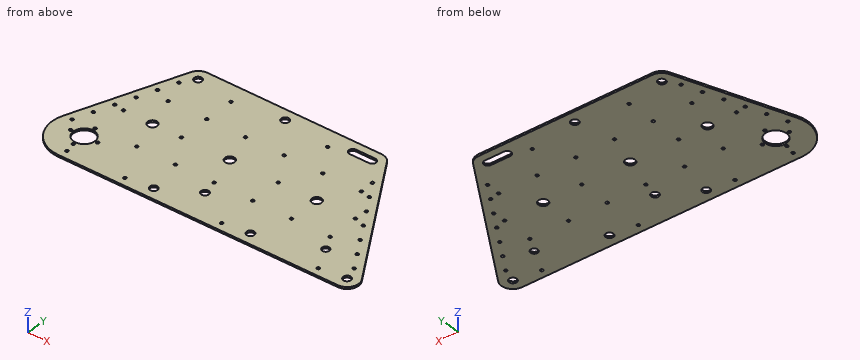
from build123d import *

# Parameters (mm, degrees)
SKETCH2_R           = 3.9998
SKETCH2_R_2         = 1.499925
SKETCH2_R_3         = 4.99975
SKETCH2_R_4         = 3.7498125
SKETCH2_R_5         = 1.5
SKETCH2_R_6         = 10.99945
BOSS_EXTRUDE1_DEPTH = 2


with BuildPart() as part:
    # Sketch2 → Boss-Extrude1 (new body)
    with BuildSketch(Plane.XY):
        with BuildLine():
            Line((96.362607148, 83.91244893), (182.746139217, -55.124360407))
            ThreePointArc((182.746139217, -55.124360407), (183.120738534, -67.267781048), (172.665833933, -73.456315551))
            Line((172.665833933, -73.456315551), (-116.301106221, -73.709344442))
            ThreePointArc((-116.301106221, -73.709344442), (-143.610306979, -59.428306601), (-147.408355202, -28.84538134))
            Line((-147.408355202, -28.84538134), (-105.239440592, 83.486872373))
            ThreePointArc((-105.239440592, 83.486872373), (-100.811651195, 88.586021375), (-94.331273913, 90.486376541))
            Line((-94.331273913, 90.486376541), (85.638662445, 90.486376541))
            ThreePointArc((85.638662445, 90.486376541), (91.93104468, 88.717175744), (96.362607148, 83.91244893))
        make_face()
        with Locations((-94.331273913, 78.486872372)):
            Circle(SKETCH2_R, mode=Mode.SUBTRACT)
        with Locations((-4.335773913, 78.486872372)):
            Circle(SKETCH2_R, mode=Mode.SUBTRACT)
        with Locations((-54.333273913, 70.986872372)):
            Circle(SKETCH2_R_2, mode=Mode.SUBTRACT)
        with Locations((-103.671855402, 65.368244598)):
            Circle(SKETCH2_R_2, mode=Mode.SUBTRACT)
        with Locations((-110.669996254, 46.632415776)):
            Circle(SKETCH2_R_2, mode=Mode.SUBTRACT)
        with Locations((-94.331273913, 39.98689418)):
            Circle(SKETCH2_R_2, mode=Mode.SUBTRACT)
        with Locations((-117.667881298, 27.897271817)):
            Circle(SKETCH2_R_2, mode=Mode.SUBTRACT)
        with Locations((-114.330273913, 7.486872372)):
            Circle(SKETCH2_R_2, mode=Mode.SUBTRACT)
        with Locations((-124.665791603, 9.162060229)):
            Circle(SKETCH2_R_2, mode=Mode.SUBTRACT)
        with Locations((-131.663765383, -9.573321299)):
            Circle(SKETCH2_R_2, mode=Mode.SUBTRACT)
        with Locations((-116.330173913, -26.513127628)):
            Circle(SKETCH2_R_2, mode=Mode.SUBTRACT)
        with Locations((-138.661805034, -28.308879181)):
            Circle(SKETCH2_R_2, mode=Mode.SUBTRACT)
        with Locations((-130.329473913, -40.513127628)):
            Circle(SKETCH2_R_2, mode=Mode.SUBTRACT)
        with Locations((-102.330873913, -40.513127628)):
            Circle(SKETCH2_R_2, mode=Mode.SUBTRACT)
        with Locations((-114.330273913, -65.013127628)):
            Circle(SKETCH2_R_2, mode=Mode.SUBTRACT)
        with Locations((-116.330173913, -54.513127628)):
            Circle(SKETCH2_R_2, mode=Mode.SUBTRACT)
        with Locations((8.663576087, -40.513127628)):
            Circle(SKETCH2_R, mode=Mode.SUBTRACT)
        with Locations((-54.333273913, -65.013127628)):
            Circle(SKETCH2_R_2, mode=Mode.SUBTRACT)
        with Locations((-27.334544722, -61.513127628)):
            Circle(SKETCH2_R, mode=Mode.SUBTRACT)
        with Locations((-74.332273913, -25.013127628)):
            Circle(SKETCH2_R_2, mode=Mode.SUBTRACT)
        with Locations((-84.331773913, 7.486872372)):
            Circle(SKETCH2_R_3, mode=Mode.SUBTRACT)
        with Locations((-54.333273913, 7.486872372)):
            Circle(SKETCH2_R_2, mode=Mode.SUBTRACT)
        with Locations((-34.334273913, -25.013127628)):
            Circle(SKETCH2_R_2, mode=Mode.SUBTRACT)
        with Locations((-54.333273913, 39.986891336)):
            Circle(SKETCH2_R_2, mode=Mode.SUBTRACT)
        with Locations((-14.335273913, 39.986886595)):
            Circle(SKETCH2_R_2, mode=Mode.SUBTRACT)
        with Locations((-4.335773913, 7.486872372)):
            Circle(SKETCH2_R_3, mode=Mode.SUBTRACT)
        with Locations((5.663726087, -25.013127628)):
            Circle(SKETCH2_R_2, mode=Mode.SUBTRACT)
        with Locations((85.659726087, -25.013127628)):
            Circle(SKETCH2_R_2, mode=Mode.SUBTRACT)
        with Locations((45.661726087, -25.013127628)):
            Circle(SKETCH2_R_2, mode=Mode.SUBTRACT)
        with Locations((45.661726087, 7.486872372)):
            Circle(SKETCH2_R_2, mode=Mode.SUBTRACT)
        with Locations((25.662726087, 39.98688375)):
            Circle(SKETCH2_R_2, mode=Mode.SUBTRACT)
        with Locations((45.661726087, 70.986872372)):
            Circle(SKETCH2_R_2, mode=Mode.SUBTRACT)
        with Locations((65.660726087, 39.986879958)):
            Circle(SKETCH2_R_2, mode=Mode.SUBTRACT)
        with Locations((72.660376087, -61.513127628)):
            Circle(SKETCH2_R, mode=Mode.SUBTRACT)
        with Locations((45.661726087, -65.013127628)):
            Circle(SKETCH2_R_2, mode=Mode.SUBTRACT)
        with Locations((125.657726087, -25.013127628)):
            Circle(SKETCH2_R_2, mode=Mode.SUBTRACT)
        with Locations((133.657326087, -40.513127628)):
            Circle(SKETCH2_R_4, mode=Mode.SUBTRACT)
        with Locations((145.656716219, -65.013127628)):
            Circle(SKETCH2_R_2, mode=Mode.SUBTRACT)
        with Locations((172.655376087, -61.513127628)):
            Circle(SKETCH2_R, mode=Mode.SUBTRACT)
        with Locations((168.349885089, -47.111508591)):
            Circle(SKETCH2_R_2, mode=Mode.SUBTRACT)
        with Locations((157.795381517, -30.123727868)):
            Circle(SKETCH2_R_2, mode=Mode.SUBTRACT)
        with Locations((147.240959183, -13.136077902)):
            Circle(SKETCH2_R_2, mode=Mode.SUBTRACT)
        with Locations((136.686149927, 3.852194828)):
            Circle(SKETCH2_R_2, mode=Mode.SUBTRACT)
        with Locations((125.657726087, 7.486872372)):
            Circle(SKETCH2_R_2, mode=Mode.SUBTRACT)
        with Locations((85.659726087, 7.486872372)):
            Circle(SKETCH2_R_3, mode=Mode.SUBTRACT)
        with Locations((126.131439072, 20.840309178)):
            Circle(SKETCH2_R_2, mode=Mode.SUBTRACT)
        with Locations((115.576938019, 37.828085844)):
            Circle(SKETCH2_R_2, mode=Mode.SUBTRACT)
        with Locations((105.658726087, 39.986878061)):
            Circle(SKETCH2_R_5, mode=Mode.SUBTRACT)
        with Locations((105.022596502, 54.815605735)):
            Circle(SKETCH2_R_2, mode=Mode.SUBTRACT)
        with Locations((-116.330173913, -40.513127628)):
            Circle(SKETCH2_R_6, mode=Mode.SUBTRACT)
        with BuildLine():
            Line((65.660726087, 82.486872372), (85.659726087, 82.486872372))
            ThreePointArc((85.659726087, 82.486872372), (89.659726087, 78.486872372), (85.659726087, 74.486872372))
            Line((85.659726087, 74.486872372), (65.660726087, 74.486872372))
            ThreePointArc((65.660726087, 74.486872372), (61.660726087, 78.486872372), (65.660726087, 82.486872372))
        make_face(mode=Mode.SUBTRACT)
    extrude(amount=BOSS_EXTRUDE1_DEPTH)


solid = part.part
Could you check a few things on this model? Use its own coordinates, in mm. Give positions to 0.01 mm unless a question says otherwise; leave off trailing zeros. Order: outer loops, then holes, each group sorted by start corner. A loop starts at its lowest first (then second) coordinate and runs counter-clockwise, first axis right, second up. Notation, with made-up numbers: M -16,29 L 6,29 A20 ccw 6,42 Z; hole C 57,40.25 d9. An arc over 180 degrees is marked long. One line per question, with ' | ' between items.
1. I want a section at C-C (y = -1.5). List the corners of the cut face in (x, z) for me.
Results:
outline: M -137.14,0 L 149.43,0 L 149.43,2 L -137.14,2 Z
2. I'm going to push a flat-ended pin straight in: pin 1 (1 mm diameter, centred on x = 134.5, z = 1.5, fed in from +Y). Where does the tip first touch, or does it pass through?
Results:
pin 1: y = 23.33
3. I want a section at A-A (x = -27). List the corners of the cut face in (y, z) for me, and give its area (3 significant figures).
Results:
outline: M -73.63,0 L -65.5,0 L -65.5,2 L -73.63,2 Z; M -57.53,0 L 90.49,0 L 90.49,2 L -57.53,2 Z | area: 312 mm²
4. If I drill on line 1 (X direction, y = -61.5, z = 0.6); line 2 (Y direction, x = -34.5, z = 0.8); line 3 (X direction, y = -43.5, z = 0.35), over which ranges is the centre line in solid material (lowest first)?
Results:
line 1: -142.05 to -31.33, -23.33 to 68.66, 76.66 to 168.66, 176.66 to 184.6 | line 2: -73.64 to -26.5, -23.52 to 90.49 | line 3: -149.39 to -126.92, -105.74 to 6, 11.32 to 131.39, 135.92 to 175.52
5. I want a section at B-B (z = 1.3). Give the number of separate pieces and of enclosed holes in the cut face, and give its area (3 significant figures).
Results:
separate pieces: 1 | enclosed holes: 51 | area: 43,300 mm²
